The listing builds one solid part. Answer for the finished solid, in the listing's coordinates (mm). Face numbers are marked on the shaded views. A direction names the side the tool comes from. Give positions to 0.01 mm unless a question says otherwise; leave off trailing zeros. Order: outer loops, then holes, each group sorted by start corner. A loop starts at its lowest first (then second) coordinate and runs counter-clockwise, first axis right, second up. Notation, with made-up numbers: (81, 26.5) - (131, 26.5) arc R20 cw to (131, 34.5) - close; hole circle Ø8 at (10, 88). An arc over 180 degrees is marked (long way). Write each question's results on one line, items separated by ' | '. Start each with the question number.
1. Find the intervals of material crossed by L1, parallel to X at y = 0.5, z = -1.4; L2, parallel to Z at x = 6, y = -5; L3, parallel to Y at x = 26, z = -0.55, in increasing order.
2. Section B-B (z = 1.75) is taken. Give the vertices of the cut face in (x, y), and give its area (3 significant figures).
3. Section C-C (x = 19) is taken. Give the vertices of the cut face in (y, z).
4. Flat-ended cylindrical pins translate along their axes: pin 1 (0.9 mm diameter, centred on x = 0, z = 1.5, fed in from +Y); pin 2 (1.2 mm diameter, centred on x = 26, y = 0, fed in from -Z); pin 3 (7.5 mm diameter, centred on x = 9.5, y = -0.5, fed in from +Z); pin 4 (2 mm diameter, centred on y = 0, z = 1.5, fed in from +X). Find the tip coordinate at first contact, or state that the pin passes through.
5. Section D-D (z = -0.65) is taken. Give the vertices of the cut face in (x, y) (3 decimals), and give its area (3 significant figures).
6. Which of the six approach directions +Z, -Z, +X, -X, +Y, -Y give full straight-line access (tool end or side, diameter ignored) to the marked faces 1 and 2?
7. Section A-A (y = 0) is taken. Give the vertices of the cut face in (x, z), and give its area (3 significant figures).
Autodesk Inventor part; units mm, degrees
ref_plane "YZ Plane" through (0, 0, 0) normal (1, 0, 0) x (0, 1, 0)
ref_plane "XZ Plane" through (0, 0, 0) normal (0, 1, 0) x (-1, 0, 0)
ref_plane "XY Plane" through (0, 0, 0) normal (0, 0, 1) x (1, 0, 0)
sketch "Szkic1" plane through (0, 0, 0) normal (0, 0, 1) x (1, 0, 0)
  circle A0 centre (0, 0) radius 7.5 construction
  line L0 (0, 7.5) -> (30, 7.5)
  line L1 (30, 7.5) -> (30, -7.5)
  line L2 (30, -7.5) -> (0, -7.5)
  line L3 (0, -7.5) -> (0, 7.5) construction
  arc A1 (0, 7.5) -> (0, -7.5) centre (0, 0) ccw
  line L4 (-1, -2) -> (1, -2)
  line L5 (1, -2) -> (1, 2)
  line L6 (1, 2) -> (-1, 2)
  line L7 (-1, 2) -> (-1, -2)
  line L8 (-1, -2) -> (1, 2) construction
  line L9 (1, -2) -> (-1, 2) construction
  circle A2 centre (26, 0) radius 4
  line L10 (-15, 0) -> (37.5, 0) construction
  line L11 (0, 7.5) -> (26.5284, 3.965)
  line L12 (0, -7.5) -> (26.5284, -3.965)
  circle A3 centre (26, 0) radius 0.75
  circle A4 centre (19, 0) radius 0.75
  point P0 (30, 0)
  dimension "d0" = 15
  dimension "d1" = 2
  dimension "d2" = 4
  dimension "d3" = 30
  dimension "d8" = 8
  dimension "d9" = 1.5
  dimension "d10" = 1.5
  dimension "d11" = 7
  dimension "d12" = 19
extrude "Wyciągnięcie proste1" add sketch "Szkic1" against normal blind 2 contours L11 A2 L12 A1 | A2 | L7 L6 L5 L4
extrude "Wyciągnięcie proste2" add sketch "Szkic1" along normal blind 3 contours L7 L6 L5 L4
fillet "Zaokrąglenie1" radius 0.6 4 edges at (-1, -2, 1.5) (1, -2, 1.5) (-1, 2, 1.5) (1, 2, 1.5)
properties part number "tweaker" material "PLA"
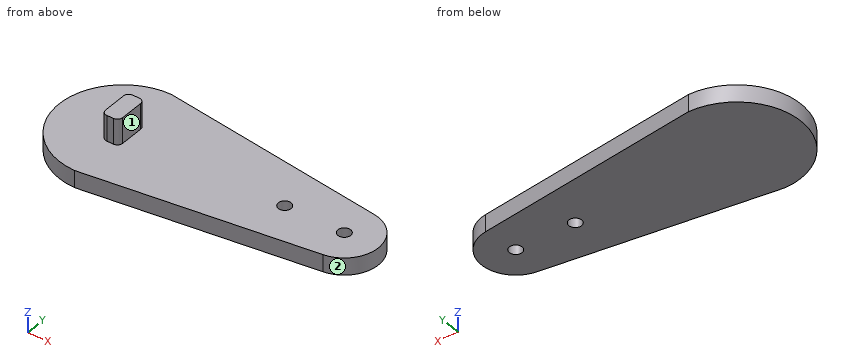
Reported:
1) L1: -7.48 to 18.44, 19.56 to 25.44, 26.56 to 29.97 | L2: -2 to 0 | L3: -4.04 to -0.75, 0.75 to 4.04
2) outline: (-1, -1.4) arc R0.6 ccw to (-0.4, -2) - (0.4, -2) arc R0.6 ccw to (1, -1.4) - (1, 1.4) arc R0.6 ccw to (0.4, 2) - (-0.4, 2) arc R0.6 ccw to (-1, 1.4) - close | area: 7.69 mm²
3) outline: (-4.97, -2) - (-0.75, -2) - (-0.75, 0) - (-4.97, 0) - close; (0.75, -2) - (4.97, -2) - (4.97, 0) - (0.75, 0) - close
4) pin 1: y = 2 | pin 2: through | pin 3: z = 0 | pin 4: x = 1
5) outline: (0, -7.5) - (26.528, -3.965) arc R4 ccw to (26.528, 3.965) - (0, 7.5) arc R7.5 ccw to start; hole circle Ø1.5 at (19, 0); hole circle Ø1.5 at (26, 0) | area: 410 mm²
6) face 1: +Z, +X, +Y, -Y | face 2: +Z, -Z, +X
7) outline: (-7.5, -2) - (18.25, -2) - (18.25, 0) - (1, 0) - (1, 3) - (-1, 3) - (-1, 0) - (-7.5, 0) - close; (19.75, -2) - (25.25, -2) - (25.25, 0) - (19.75, 0) - close; (26.75, -2) - (30, -2) - (30, 0) - (26.75, 0) - close | area: 75.0 mm²
